```python
from build123d import *

# Parameters (mm, degrees)
F0_R     = 2
F1_DEPTH = 1.5


with BuildPart() as f1:
    # F0 (on Top) → F1 (new body, symmetric)
    with BuildSketch(Plane.XY):
        Polygon((3, 29.24), (-27.8, 29.24), (-31, 29.24), (-31, 20.24), (-27.8, 20.24), (-27.8, 11.24), (-31, 11.24), (-31, 2.237353), (-27.8, 2.237353), (-27.8, -19.5), (-27.8, -29.235), (3, -29.24), (3, -19.5), (3, 19.5), align=None)
        with Locations((-20.85, -24.375)):
            Circle(F0_R, mode=Mode.SUBTRACT)
        with Locations((-20.85, -19.5)):
            Circle(F0_R, mode=Mode.SUBTRACT)
        with Locations((-20.85, -14.625)):
            Circle(F0_R, mode=Mode.SUBTRACT)
        with Locations((-20.85, -9.75)):
            Circle(F0_R, mode=Mode.SUBTRACT)
        with Locations((-20.85, -4.875)):
            Circle(F0_R, mode=Mode.SUBTRACT)
        with Locations((-20.85, 0)):
            Circle(F0_R, mode=Mode.SUBTRACT)
        with Locations((-13.9, -24.375)):
            Circle(F0_R, mode=Mode.SUBTRACT)
        with Locations((-6.95, -24.375)):
            Circle(F0_R, mode=Mode.SUBTRACT)
        with Locations((-13.9, -19.5)):
            Circle(F0_R, mode=Mode.SUBTRACT)
        with Locations((-13.9, -14.625)):
            Circle(F0_R, mode=Mode.SUBTRACT)
        with Locations((-6.95, -19.5)):
            Circle(F0_R, mode=Mode.SUBTRACT)
        with Locations((-6.95, -14.625)):
            Circle(F0_R, mode=Mode.SUBTRACT)
        with Locations((0, -24.375)):
            Circle(F0_R, mode=Mode.SUBTRACT)
        with Locations((0, -19.5)):
            Circle(F0_R, mode=Mode.SUBTRACT)
        with Locations((0, -14.625)):
            Circle(F0_R, mode=Mode.SUBTRACT)
        with Locations((-13.9, -9.75)):
            Circle(F0_R, mode=Mode.SUBTRACT)
        with Locations((-6.95, -9.75)):
            Circle(F0_R, mode=Mode.SUBTRACT)
        with Locations((-13.9, -4.875)):
            Circle(F0_R, mode=Mode.SUBTRACT)
        with Locations((-13.9, 0)):
            Circle(F0_R, mode=Mode.SUBTRACT)
        with Locations((-6.95, -4.875)):
            Circle(F0_R, mode=Mode.SUBTRACT)
        with Locations((-6.95, 0)):
            Circle(F0_R, mode=Mode.SUBTRACT)
        with Locations((0, -9.75)):
            Circle(F0_R, mode=Mode.SUBTRACT)
        with Locations((0, -4.875)):
            Circle(F0_R, mode=Mode.SUBTRACT)
        Circle(F0_R, mode=Mode.SUBTRACT)
        with Locations((-20.85, 4.875)):
            Circle(F0_R, mode=Mode.SUBTRACT)
        with Locations((-20.85, 9.75)):
            Circle(F0_R, mode=Mode.SUBTRACT)
        with Locations((-20.85, 14.625)):
            Circle(F0_R, mode=Mode.SUBTRACT)
        with Locations((-20.85, 19.5)):
            Circle(F0_R, mode=Mode.SUBTRACT)
        with Locations((-20.85, 24.375)):
            Circle(F0_R, mode=Mode.SUBTRACT)
        with Locations((-13.9, 4.875)):
            Circle(F0_R, mode=Mode.SUBTRACT)
        with Locations((-6.95, 4.875)):
            Circle(F0_R, mode=Mode.SUBTRACT)
        with Locations((-13.9, 9.75)):
            Circle(F0_R, mode=Mode.SUBTRACT)
        with Locations((-6.95, 9.75)):
            Circle(F0_R, mode=Mode.SUBTRACT)
        with Locations((0, 4.875)):
            Circle(F0_R, mode=Mode.SUBTRACT)
        with Locations((0, 9.75)):
            Circle(F0_R, mode=Mode.SUBTRACT)
        with Locations((-13.9, 14.625)):
            Circle(F0_R, mode=Mode.SUBTRACT)
        with Locations((-13.9, 19.5)):
            Circle(F0_R, mode=Mode.SUBTRACT)
        with Locations((-6.95, 14.625)):
            Circle(F0_R, mode=Mode.SUBTRACT)
        with Locations((-6.95, 19.5)):
            Circle(F0_R, mode=Mode.SUBTRACT)
        with Locations((-13.9, 24.375)):
            Circle(F0_R, mode=Mode.SUBTRACT)
        with Locations((-6.95, 24.375)):
            Circle(F0_R, mode=Mode.SUBTRACT)
        with Locations((0, 14.625)):
            Circle(F0_R, mode=Mode.SUBTRACT)
        with Locations((0, 19.5)):
            Circle(F0_R, mode=Mode.SUBTRACT)
        with Locations((0, 24.375)):
            Circle(F0_R, mode=Mode.SUBTRACT)
    extrude(amount=F1_DEPTH, both=True)


solid = f1.part
```
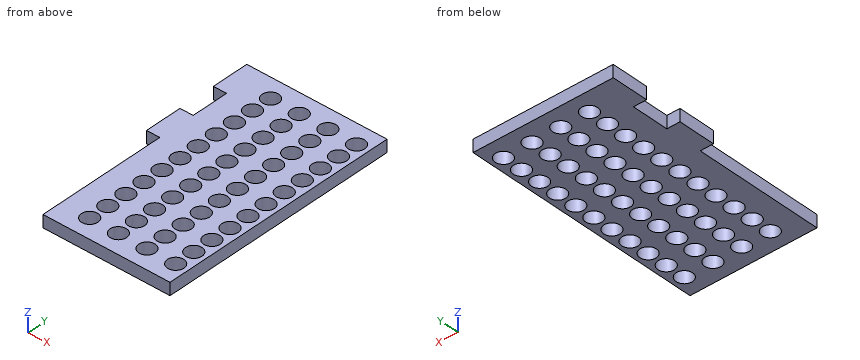
Design review of the part built by this model. Coordinates are the model's own, in mm. Coordinates: 2 decimals unless noted, no trailing zeros. Order: outer loops, then holes, each group sorted by start corner. A loop starts at its lowest first (then second) coordinate and runs counter-clockwise, first axis right, second up. Notation, with made-up numbers: M 44.5,85.25 L 50.5,85.25 A19 ccw 50.5,96.25 Z; hole C -0.5,80 d6. An arc over 180 degrees is marked long. Answer as a JSON object with one key per item and string values. Group by question number.
1) Add section A-A, the plane x = -29. Write out the cut boundary in (y, z).
2) For pin 1 (1.5 mm diameter, centred on y = -15.5, z = -1, fed in from -X), flat-tipped, find the tip position at first contact; note if it passes through.
3) Add section C-C, the plane x = -14.5. Count the separate pieces of the cut face and the enclosed holes in it, then the cut area to 3 significant figures.
4) Wall thickness on L1, parallel to X at y = -5, z = -0.6; L2, parallel to X at y = 5.5, z = -0.5; L3, parallel to Y at x = -29, z = 0: over which ranges is each line inside the solid? List them lowest first.
5) Add section B-B, the plane y = 9.75. Write out the cut boundary in (x, z), then the cut area to 3 significant figures.
Computed values:
{
 "1": {"outline": "M 2.24,-1.5 L 11.24,-1.5 L 11.24,1.5 L 2.24,1.5 Z; M 20.24,-1.5 L 29.24,-1.5 L 29.24,1.5 L 20.24,1.5 Z"},
 "2": {"pin 1": "stops at x = -27.8"},
 "3": {"separate pieces": "12", "enclosed holes": "0", "area": "49.5 mm^2"},
 "4": {"L1": "x = -27.8 to -22.85, -18.85 to -15.9, -11.9 to -8.95, -4.95 to -2, 2 to 3", "L2": "x = -31 to -22.75, -18.95 to -15.8, -12 to -8.85, -5.05 to -1.9, 1.9 to 3", "L3": "y = 2.24 to 11.24, 20.24 to 29.24"},
 "5": {"outline": "M -31,-1.5 L -22.85,-1.5 L -22.85,1.5 L -31,1.5 Z; M -18.85,-1.5 L -15.9,-1.5 L -15.9,1.5 L -18.85,1.5 Z; M -11.9,-1.5 L -8.95,-1.5 L -8.95,1.5 L -11.9,1.5 Z; M -4.95,-1.5 L -2,-1.5 L -2,1.5 L -4.95,1.5 Z; M 2,-1.5 L 3,-1.5 L 3,1.5 L 2,1.5 Z", "area": "54.0 mm^2"}
}
